```python
from build123d import *

# Parameters (mm, degrees)
BOSS_EXTRUDE1_DEPTH      = 2.3876
BOSS_EXTRUDE1_DEPTH_BACK = 2.3876
SKETCH4_R                = 3.2639
CUT_EXTRUDE1_DEPTH       = 5.7752
SKETCH7_W                = 101.6
SKETCH7_H                = 101.6
BOSS_EXTRUDE2_DEPTH      = 4.7752
SKETCH10_R               = 4.191
CUT_EXTRUDE3_DEPTH       = 5.7752
SKETCH11_OUTSIDE_W       = 132.352
SKETCH11_OUTSIDE_H       = 132.352
SKETCH11_OUTSIDE_W_2     = 101.6
SKETCH11_OUTSIDE_H_2     = 71.12
CUT_EXTRUDE4_DEPTH       = 4.7752


with BuildPart() as part:
    # Sketch3 → Boss-Extrude1 (new body, two sides)
    with BuildSketch(Plane.XY) as boss_extrude1_sk:
        Polygon((50.8, -25.4), (50.8, -50.8), (-50.8, -50.8), (-50.8, 50.8), (-25.4, 50.8), align=None)
    extrude(amount=BOSS_EXTRUDE1_DEPTH)
    extrude(boss_extrude1_sk.sketch, amount=-BOSS_EXTRUDE1_DEPTH_BACK)

    # Sketch4 → Cut-Extrude1 (cut, through all)
    with BuildSketch(Plane.XY.offset(2.3876)):
        with Locations((-38.1, -38.1)):
            Circle(SKETCH4_R)
        with Locations((-12.7, -38.1)):
            Circle(SKETCH4_R)
        with Locations((12.7, -38.1)):
            Circle(SKETCH4_R)
        with Locations((-38.1, -12.7)):
            Circle(SKETCH4_R)
        with Locations((-38.1, 12.7)):
            Circle(SKETCH4_R)
        with Locations((38.1, -38.1)):
            Circle(SKETCH4_R)
        with Locations((-38.1, 38.1)):
            Circle(SKETCH4_R)
    extrude(amount=-CUT_EXTRUDE1_DEPTH, mode=Mode.SUBTRACT)

    # Sketch7 → Boss-Extrude2 (add)
    with BuildSketch(Plane.XY.offset(2.3876)):
        Rectangle(SKETCH7_W, SKETCH7_H)
    extrude(amount=-BOSS_EXTRUDE2_DEPTH)

    # Sketch10 → Cut-Extrude3 (cut, through all)
    with BuildSketch(Plane.XY.offset(2.3876)):
        with Locations((-33.02, 0)):
            Circle(SKETCH10_R)
        with Locations((33.02, 0)):
            Circle(SKETCH10_R)
        with Locations((0, 25.4)):
            Circle(SKETCH10_R)
        with Locations((0, -25.4)):
            Circle(SKETCH10_R)
    extrude(amount=-CUT_EXTRUDE3_DEPTH, mode=Mode.SUBTRACT)

    # Sketch11 outside → Cut-Extrude4 (cut)
    with BuildSketch(Plane.XY.offset(2.3876)):
        Rectangle(SKETCH11_OUTSIDE_W, SKETCH11_OUTSIDE_H)
        Rectangle(SKETCH11_OUTSIDE_W_2, SKETCH11_OUTSIDE_H_2, mode=Mode.SUBTRACT)
    extrude(amount=-CUT_EXTRUDE4_DEPTH, mode=Mode.SUBTRACT)


solid = part.part
```
Geometry check sheet. Reference: the model listing, model coordinates, mm. Coordinates: 2 decimals unless noted, no trailing zeros. Loops run counter-clockwise (first coordinate to the right, second up) from the corner with the lowest first, then second, coordinate; pieces in that order, holes last.
Item 1: Sectioned sample at A-A, the plane y = 0. Record the boundary of the cut face in (x, z).
Item 2: Sectioned sample at D-D, the plane y = 25.4. Record the boundary of the cut face in (x, z).
Item 3: Release check for a two-part mould opening along Y. For faces 1 (the face through (-0.546, -21.245, 0.033)), 2 (the face through (-1, -35.56, 0)), 3 (the face through (-36.346, -2.55, 0.033)), 4 (the face through (-50.8, 0, 0)) record: released by +Y, released by -Y, zero draft, split by the parting line, or undercut.
Item 4: Sectioned sample at B-B, the plane x = -33.02. Record the boundary of the cut face in (y, z).
Item 5: Sectioned sample at C-C, the plane x = 0. Record the boundary of the cut face in (y, z), then the cut area to 3 significant figures.
Item 6: Thickness scan on line 1 (Y direction, x = 0, z = 1); line 2 (X direction, y = -3, z = 0.2); line 3 (Y direction, x = -33.02, z = 0.9). Record the ranges inside material, lowest first.
Check result:
1. outline: (-50.8, -2.39) - (-37.21, -2.39) - (-37.21, 2.39) - (-50.8, 2.39) - close; (-28.83, -2.39) - (28.83, -2.39) - (28.83, 2.39) - (-28.83, 2.39) - close; (37.21, -2.39) - (50.8, -2.39) - (50.8, 2.39) - (37.21, 2.39) - close
2. outline: (-50.8, -2.39) - (-4.19, -2.39) - (-4.19, 2.39) - (-50.8, 2.39) - close; (4.19, -2.39) - (50.8, -2.39) - (50.8, 2.39) - (4.19, 2.39) - close
3. face 1: undercut
3. face 2: released by -Y
3. face 3: undercut
3. face 4: zero draft
4. outline: (-35.56, -2.39) - (-4.19, -2.39) - (-4.19, 2.39) - (-35.56, 2.39) - close; (4.19, -2.39) - (35.56, -2.39) - (35.56, 2.39) - (4.19, 2.39) - close
5. outline: (-35.56, -2.39) - (-29.59, -2.39) - (-29.59, 2.39) - (-35.56, 2.39) - close; (-21.21, -2.39) - (21.21, -2.39) - (21.21, 2.39) - (-21.21, 2.39) - close; (29.59, -2.39) - (35.56, -2.39) - (35.56, 2.39) - (29.59, 2.39) - close
5. area: 260 mm2
6. line 1: y = -35.56 to -29.59, -21.21 to 21.21, 29.59 to 35.56
6. line 2: x = -50.8 to -35.95, -30.09 to 30.09, 35.95 to 50.8
6. line 3: y = -35.56 to -4.19, 4.19 to 35.56
